Input: dimensioned drawing with shaded views. Units: mm. Origin: part minimum x, y, z. A direction names the side the tool comes from. Coordinates: 2 decimals unless noted, no trailing zeros. Loops run counter-clockwise (first coordinate to the right, second up) from the corner with the lowest first, then second, coordinate; pieces in that order, holes last.
Item 1: Contact query for flat-ended pins moving along their axis: P1, Ø5, axis at y = 10, z = 6, coming from the +X side; P2, Ø1, axis at x = 34, z = 2, coming from the -Y side; P3, Ø1.8, axis at y = 9.5, z = 4, coming from the -X side. Output: stop coordinate, or through.
Item 2: Ray query, line 1 along Y through (x, z) = (43.5, 6.5); line 2 along Z through (x, y) = (7.5, 87); line 3 along Y through (x, z) = (17, 3.75). Return the intervals inside material, ascending.
Item 3: Reachability of the marked faces 1, 2 and 3 from +Z, -Z, +X, -X, +Y, -Y: full face, straight path, thin tool, end or side. Return the list, or none.
Item 4: Section B-B on y = 60. Return loops of the section in (x, z).
Item 5: Section D-D on x = 43.5. Return loops of the section in (y, z).
Item 6: Section C-C on x = 36.5. Return loops of the section in (y, z), and give its area (3 significant figures).
Item 7: Pull-direction query (Y, two-part tool) for the marked faces 4, 5 and 6; classes: released by +Y, released by -Y, zero draft, split by the parting line, or undercut.
Item 8: Section A-A on z = 4.5. Give the number of separate pieces and of enclosed holes in the cut face, and give its area (3 significant figures).
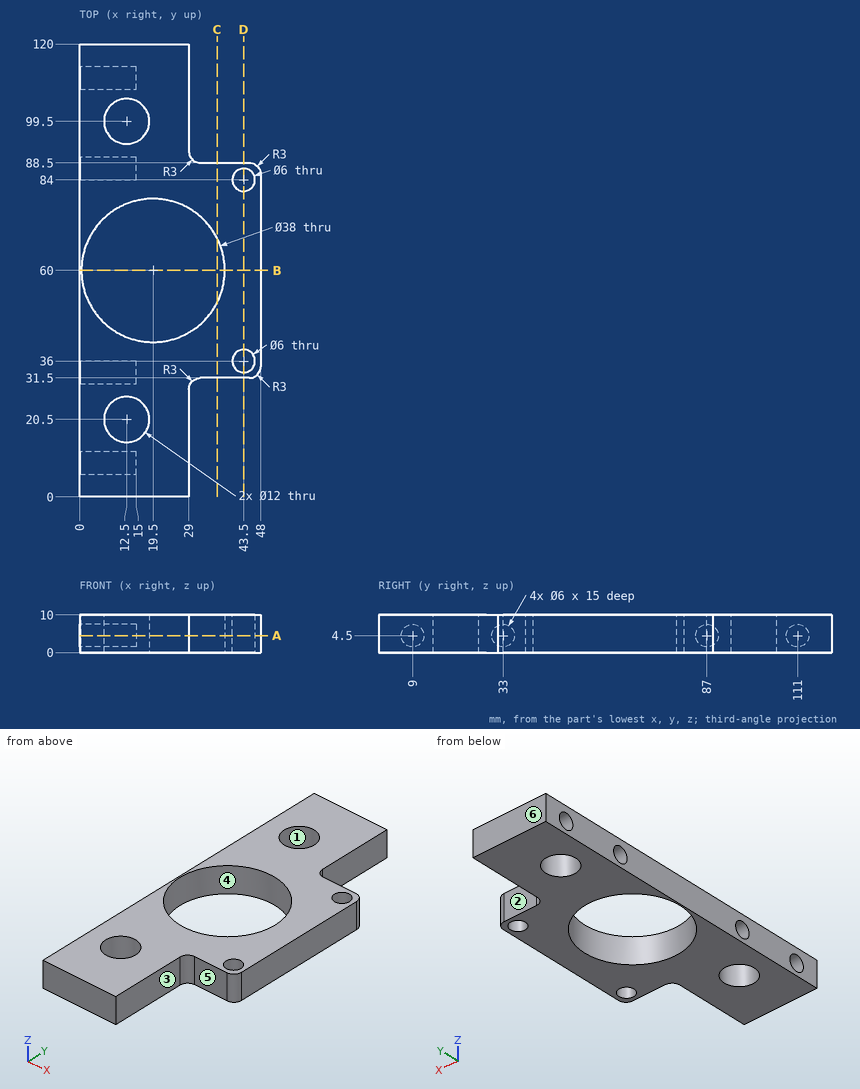
Results found:
1. P1: stops at x = 29
1. P2: stops at y = 31.5
1. P3: stops at x = 15
2. line 1: y = 31.5 to 33, 39 to 81, 87 to 88.5
2. line 2: z = 0 to 1.5, 7.5 to 10
2. line 3: y = 0 to 16.53, 24.47 to 41.17, 78.83 to 95.53, 103.47 to 120
3. face 1: +Z, -Z
3. face 2: +Z, -Z, +X, +Y
3. face 3: +Z, -Z, +X, -Y
4. outline: (0, 0) - (0.5, 0) - (0.5, 10) - (0, 10) - close; (38.5, 0) - (48, 0) - (48, 10) - (38.5, 10) - close
5. outline: (31.5, 0) - (33, 0) - (33, 10) - (31.5, 10) - close; (39, 0) - (81, 0) - (81, 10) - (39, 10) - close; (87, 0) - (88.5, 0) - (88.5, 10) - (87, 10) - close
6. outline: (31.5, 0) - (51.51, 0) - (51.51, 10) - (31.5, 10) - close; (68.49, 0) - (88.5, 0) - (88.5, 10) - (68.49, 10) - close
6. area: 400 mm2
7. face 4: undercut
7. face 5: released by -Y
7. face 6: released by +Y
8. separate pieces: 1
8. enclosed holes: 5
8. area: 2,790 mm2
